Design review of the part built by this model. Coordinates are the model's own, in mm. Face numbers are marked on the shaded views. A direction names the side the tool comes from. Give positions to 0.01 mm unless a question says otherwise; leave off trailing zeros. Order: outer loops, then holes, each group sorted by start corner. A loop starts at its lowest first (then second) coordinate and runs counter-clockwise, first axis right, second up. Notation, with made-up numbers: (26, -26.5) -> (61, -26.5) arc R14 ccw to (61, -22.5) -> close; hole circle Ø6 at (52, -25). An arc over 180 degrees is marked (long way). One line per item, written item: value. Start each with the question number.
1) Consider section B-B (z = 6.5). State the section outline as (x, y) points.
2) Tool access review of the marked faces 4, 5 and 6: name each direction out of +Z, -Z, +X, -X, +Y, -Y from which nothing blocks a thin tool from reaching the whole face with its end or side.
3) Wall thickness on line 1 along X through (y, z) = (24.5, 26.5); line 2 along X through (y, z) = (-22.5, 13.5); line 3 along Y through (x, z) = (43.5, 19): over which ranges is each line inside the solid? List them lowest first. Write a range as from..to.
4) Consider section C-C (x = 108). State the section outline as (y, z) points, plus the area to 3 significant figures.
5) The part is to be moulded in two halves that separate along Y. For the marked faces 1, 2 and 3, say which applies: released by +Y, released by -Y, zero draft, split by the parting line, or undercut.
6) Consider section D-D (x = 16). State the section outline as (y, z) points.
7) Consider section A-A (y = 0). State the section outline as (x, z) points, plus the area to 3 significant figures.
8) For pin 1 (2 mm diameter, centred on x = 128.5, z = 26.5, fed in from -Y); pin 2 (11.5 mm diameter, centred on x = 58.5, z = 11.5, fed in from -Y); pin 3 (10 mm diameter, centred on y = 17.5, z = 18.5, fed in from +X), all flat-tipped, find the tip position at first contact; note any pin that passes through.
from build123d import *

# Parameters (mm, degrees)
F0_R     = 12.7
F1_DEPTH = 12.7
F2_DEPTH = 76.2
F3_DEPTH = 25.4


with BuildPart() as f1:
    # F0 (on Top) → F1 (new body)
    with BuildSketch(Plane.XY):
        with BuildLine():
            ThreePointArc((0, 50.8), (-50.8, 0), (0, -50.8))
            Line((0, -50.8), (101.6, -50.8))
            ThreePointArc((101.6, -50.8), (152.4, 0), (101.6, 50.8))
            Line((101.6, 50.8), (0, 50.8))
        make_face()
        Circle(F0_R, mode=Mode.SUBTRACT)
        with Locations((101.6, 0)):
            Circle(F0_R, mode=Mode.SUBTRACT)
    extrude(amount=F1_DEPTH)

    # F2 (cut): a face of the model
    f2_faces = [f1.faces().sort_by_distance(p)[0] for p in [
        (50.8, -50.8, 6.35),
    ]]
    extrude(f2_faces, amount=-F2_DEPTH, mode=Mode.SUBTRACT)

    # F3 (add): a face of the model
    f3_faces = [f1.faces().sort_by_distance(p)[0] for p in [
        (150.1281549349, 0, 12.7),
    ]]
    extrude(f3_faces, amount=F3_DEPTH)


solid = f1.part
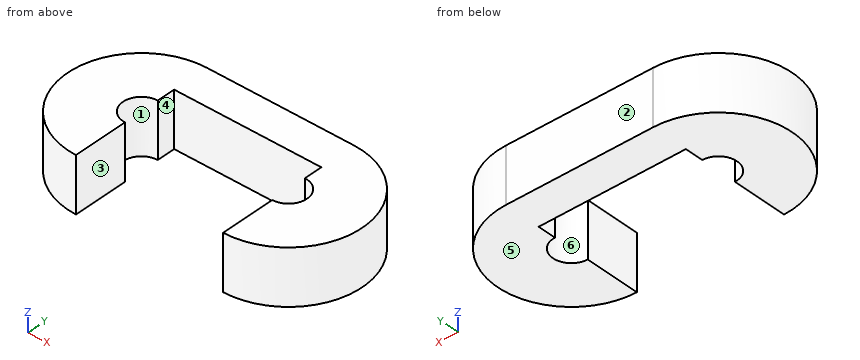
Checked values:
1. outline: (0, -50.8) -> (0, -12.7) arc R12.7 cw to (0, 12.7) -> (0, 25.4) -> (101.6, 25.4) -> (101.6, 12.7) arc R12.7 cw to (101.6, -12.7) -> (101.6, -50.8) arc R50.8 ccw to (101.6, 50.8) -> (0, 50.8) arc R50.8 ccw to start
2. face 4: +Z, -Z, -Y
2. face 5: -Z, +X, -X, +Y, -Y
2. face 6: +Z, -Z
3. line 1: x = -44.5..0, 101.6..146.1
3. line 2: x = -45.55..0, 101.6..147.15
3. line 3: y = 25.4..50.8
4. outline: (-50.4, 0) -> (-10.97, 0) -> (-10.97, 38.1) -> (-50.4, 38.1) -> close; (10.97, 0) -> (50.4, 0) -> (50.4, 38.1) -> (10.97, 38.1) -> close
4. area: 3,000 mm^2
5. face 1: undercut
5. face 2: released by +Y
5. face 3: zero draft
6. outline: (25.4, 0) -> (50.8, 0) -> (50.8, 38.1) -> (25.4, 38.1) -> close
7. outline: (-50.8, 0) -> (-12.7, 0) -> (-12.7, 38.1) -> (-50.8, 38.1) -> close; (114.3, 0) -> (152.4, 0) -> (152.4, 38.1) -> (114.3, 38.1) -> close
7. area: 2,900 mm^2
8. pin 1: stops at y = -43.7
8. pin 2: stops at y = 25.4
8. pin 3: stops at x = 150.84
